For this review, take the finished solid that the model builds, in its own axes (mm). A direction names the side the tool comes from. Give positions to 0.01 mm unless a question says otherwise; leave off trailing zeros. Order: outer loops, then holes, each group sorted by start corner. A loop starts at its lowest first (then second) coordinate and runs counter-clockwise, first axis right, second up. Notation, with made-up numbers: (18.5, -30) - (35.5, -30) arc R30 cw to (35.5, -6) - close; hole circle Ø7 at (-21.75, 29). An arc over 180 degrees is marked (long way). Use a Markdown table: item, result. Add a question column.
1) We need section A-A on x = 1. Write out the cut boundary in (y, z) (3 decimals).
2) Clearance check with flat-ended pins moving along their axes: P1, Ø1, axis at x = 1.5, z = -23.5, coming from the +Y side; P2, Ø1, axis at x = 3, z = 25, coming from the -Y side; P3, Ø3, axis at x = 4, z = 30, coming from the -Y side (3 decimals). State where each tip first meets the part, or that it passes through.
3) We need section B-B on z = -30. Write out the cut boundary in (x, y) (3 decimals).
4) Wall thickness on L1, parallel to Y at x = 2.25, z = 28 (3 decimals); L2, parallel to Y at x = 1.5, z = -21; L3, parallel to Z at x = 2.25, y = 31: over which ranges is each line inside the solid? List them lowest first.
5) We need section C-C on z = -7.5. Write out the cut boundary in (x, y).
6) Machinability: for faces 1 (the face through (3, 22.225, -33)), 2 (the face through (3, -22.225, 33)), 3 (the face through (3, -22.225, -32)), which of the approach directions +Z, -Z, +X, -X, +Y, -Y give a long, thin tool a straight path to every point of the face, cutting with its end or side? Answer none if there is none.
```python
from build123d import *

# Parameters (mm, degrees)
BOSS_EXTRUDE1_DEPTH = 6.35


with BuildPart() as part:
    # Sketch1 → Boss-Extrude1 (new body)
    with BuildSketch(Plane(origin=(0, 0, 0), x_dir=(0, 0, -1), z_dir=(1, 0, 0))):
        with BuildLine():
            ThreePointArc((-26.940768363, 22.225), (-34.925, 0), (-26.940768363, -22.225))
            Line((-26.940768363, -22.225), (26.940768363, -22.225))
            ThreePointArc((26.940768363, -22.225), (32.868388766, -11.807821347), (34.925, 0))
            ThreePointArc((34.925, 0), (32.868388766, 11.807821347), (26.940768363, 22.225))
            Line((26.940768363, 22.225), (-26.940768363, 22.225))
        make_face()
        with BuildLine():
            Line((-38.1, 22.225), (-38.1, -22.225))
            Line((-38.1, -22.225), (-26.940768363, -22.225))
            ThreePointArc((-26.940768363, -22.225), (-34.925, 0), (-26.940768363, 22.225))
            Line((-26.940768363, 22.225), (-38.1, 22.225))
        make_face()
        with BuildLine():
            ThreePointArc((26.940768363, 22.225), (0, 34.925), (-26.940768363, 22.225))
            Line((-26.940768363, 22.225), (26.940768363, 22.225))
        make_face()
        with BuildLine():
            ThreePointArc((34.925, 0), (32.868388766, -11.807821347), (26.940768363, -22.225))
            Line((26.940768363, -22.225), (38.1, -22.225))
            Line((38.1, -22.225), (38.1, 22.225))
            Line((38.1, 22.225), (26.940768363, 22.225))
            ThreePointArc((26.940768363, 22.225), (32.868388766, 11.807821347), (34.925, 0))
        make_face()
        with BuildLine():
            Line((26.940768363, -22.225), (-26.940768363, -22.225))
            ThreePointArc((-26.940768363, -22.225), (0, -34.925), (26.940768363, -22.225))
        make_face()
    extrude(amount=BOSS_EXTRUDE1_DEPTH)


solid = part.part
```
Checked values:
| question | item | result |
|---|---|---|
| 1 | outline | (-22.225, -38.1) - (22.225, -38.1) - (22.225, -26.941) arc R34.925 ccw to (22.225, 26.941) - (22.225, 38.1) - (-22.225, 38.1) - (-22.225, 26.941) arc R34.925 ccw to (-22.225, -26.941) - close |
| 2 | P1 | y = 26.28 |
| 2 | P2 | y = -24.89 |
| 2 | P3 | y = -22.225 |
| 3 | outline | (0, -22.225) - (6.35, -22.225) - (6.35, 22.225) - (0, 22.225) - close |
| 4 | L1 | -22.225 to 22.225 |
| 4 | L2 | -27.91 to 27.91 |
| 4 | L3 | -16.09 to 16.09 |
| 5 | outline | (0, -34.11) - (6.35, -34.11) - (6.35, 34.11) - (0, 34.11) - close |
| 6 | face 1 | -Z, +X, -X, +Y |
| 6 | face 2 | +Z, +X, -X, -Y |
| 6 | face 3 | -Z, +X, -X, -Y |
